Design review of the part shown in the three views and the two pictorial views. Dimensions are in mm from the part's minimum x, y and z. Coordinates: 2 decimals unless noted, no trailing zeros. Loops run counter-clockwise (first coordinate to the right, second up) from the corner with the lowest first, then second, coordinate; pieces in that order, holes last.
Q1. Add section C-C on x = 0.7. Give the boundary of the cut face in (y, z).
Q2. Add section A-A on y = 0.75. Give the boundary of the cut face in (x, z).
Q3. Wall thickness on probe 1 along Y at (x, z) = (1.85, 0.1) (1 decimal); probe 2 along Y at (x, z) = (1.2, 0.1) (1 decimal); probe 3 along X at (y, z) = (4.75, 0.1): over which ranges is each line inside the solid? List them lowest first.
Q4. Add section D-D on y = 6.5. Give the boundary of the cut face in (x, z).
Q5. Add section B-B on z = 0.1. Give the boundary of the cut face in (x, y).
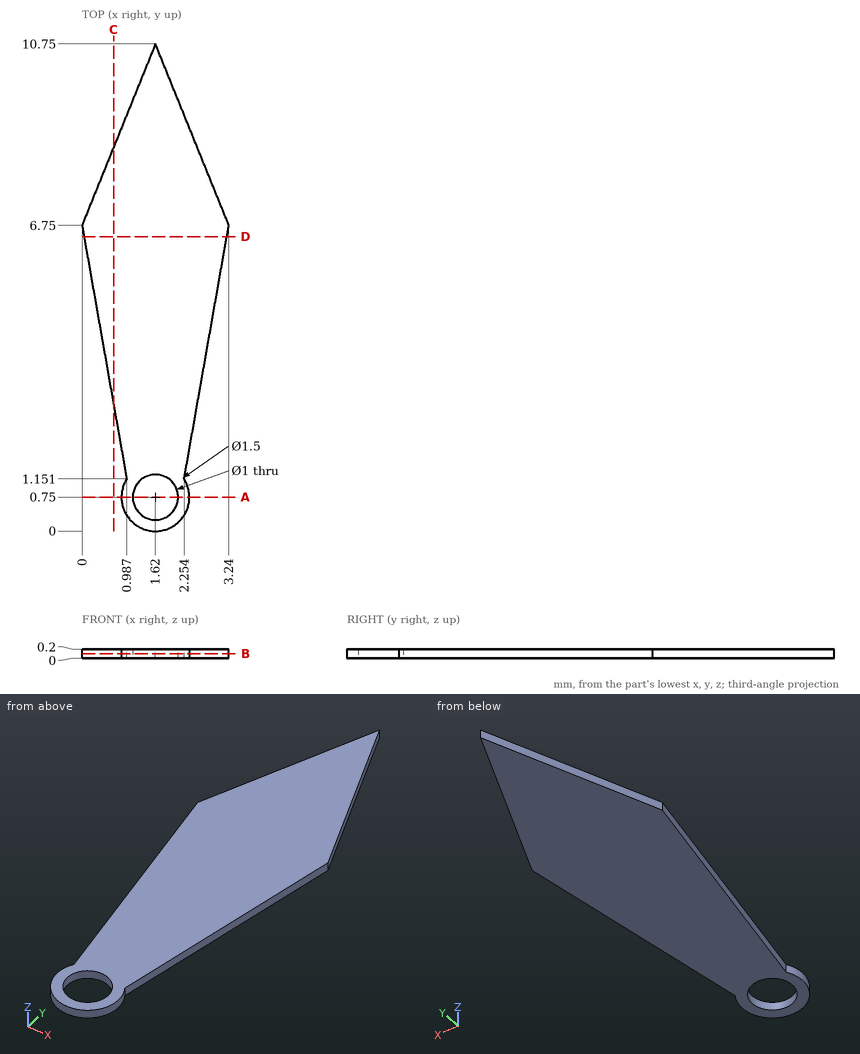
Entries:
1. outline: (2.78, 0) - (8.48, 0) - (8.48, 0.2) - (2.78, 0.2) - close
2. outline: (0.87, 0) - (1.12, 0) - (1.12, 0.2) - (0.87, 0.2) - close; (2.12, 0) - (2.37, 0) - (2.37, 0.2) - (2.12, 0.2) - close
3. probe 1: y = 0 to 0.3, 1.2 to 10.2
3. probe 2: y = 0.1 to 0.5, 1 to 9.7
3. probe 3: x = 0.35 to 2.89
4. outline: (0.04, 0) - (3.2, 0) - (3.2, 0.2) - (0.04, 0.2) - close
5. outline: (0, 6.75) - (0.99, 1.15) arc R0.75 ccw (long way) to (2.25, 1.15) - (3.24, 6.75) - (1.62, 10.75) - close; hole circle Ø1 at (1.62, 0.75)
